Check sheet for the drawn part. Datum: minimum x, y, z corner. Units: mm. A direction names the side the tool comes from. Coordinates: 2 decimals unless noted, no trailing zeros. Loops run counter-clockwise (first coordinate to the right, second up) from the corner with the lowest first, then second, coordinate; pieces in that order, holes last. Notation, with made-up numbers: (-23, 35) -> (-15, 35) arc R11 cw to (-15, 51) -> close; hole circle Ø8 at (41.5, 70.5). An arc over 180 degrees is marked (long way). Use CSV: the item, a comma, the result in double quotes. Start each with the question number.
1. Thickness scan on L1, parallel to Z at x = 54.5, y = 2.55; L2, parallel to X at y = 4.35, z = 31; L3, parallel to X at y = 2.9, z = 48. Record the ranges inside material, lowest first.
2. Sectioned sample at A-A, the plane x = 32.3. Record the cut outline in (y, z).
3. Set-up check for the marked faces 1, 2 and 3: record each of +Z, -Z, +X, -X, +Y, -Y from which the full face is reachable in a straight line by a thin tool's end or side.
4. Sectioned sample at B-B, the plane x = 54.5. Record the cut outline in (y, z).
5. Sectioned sample at D-D, the plane z = 12.5. Record the cut outline in (x, y).
6. Gauge pin test, flat ends, axial feed: pin 1 (2 mm diameter, centred on x = 48, y = 1, fed in from -Z); pin 2 (3 mm diameter, centred on x = 12.5, y = 2, fed in from +Z); pin 3 (1 mm diameter, centred on y = 4, z = 15, fed in from -X). Record the tip position at first contact, or that the pin passes through.
7. Sectioned sample at C-C, the plane y = 3.7. Record the cut outline in (x, z).
8. Release check for a two-part mould opening along Z. For the marked faces 4, 5 and 6 record: pulls with the +Z half, pulls with the -Z half, needs draft (parallel to the pull), parting line crosses it, or undercut.
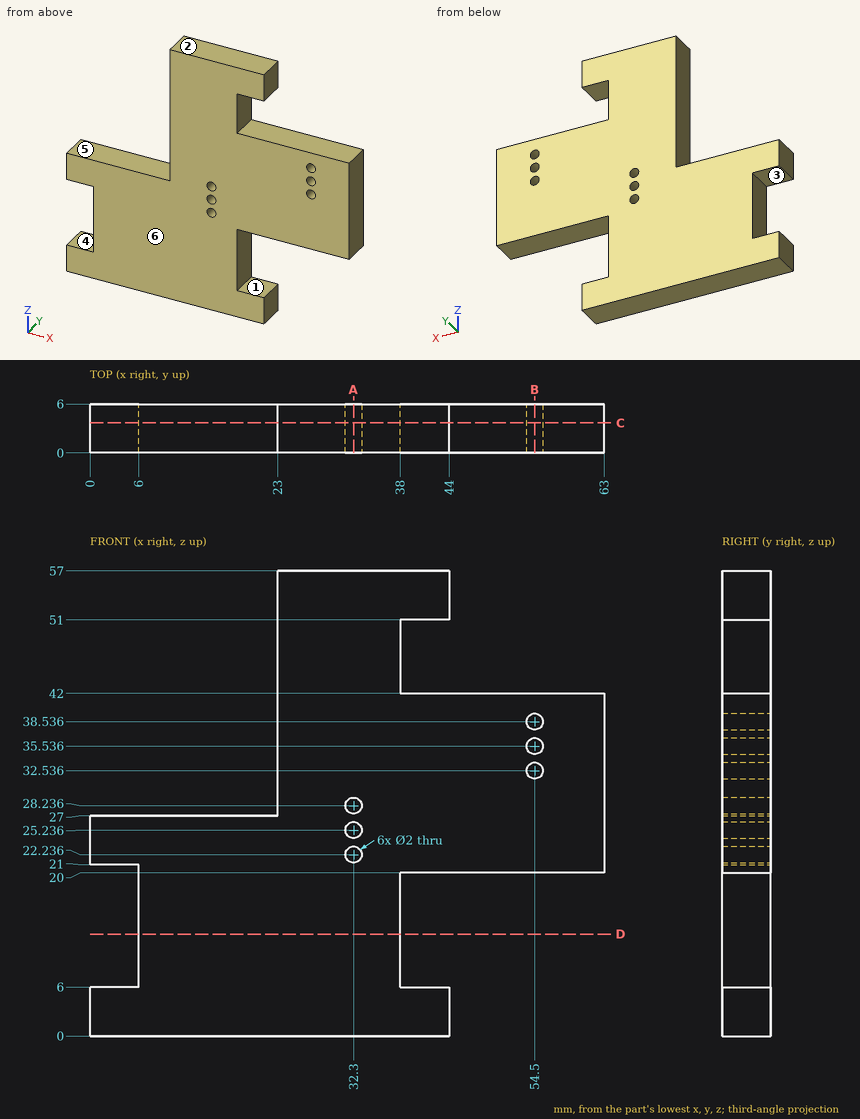
Completed:
1,L1,"20 to 31.54, 33.54 to 34.54, 36.54 to 37.54, 39.54 to 42"
1,L2,"23 to 63"
1,L3,"23 to 38"
2,outline,"(0, 0) -> (6, 0) -> (6, 21.24) -> (0, 21.24) -> close; (0, 23.24) -> (6, 23.24) -> (6, 24.24) -> (0, 24.24) -> close; (0, 26.24) -> (6, 26.24) -> (6, 27.24) -> (0, 27.24) -> close; (0, 29.24) -> (6, 29.24) -> (6, 57) -> (0, 57) -> close"
3,face 1,"+X, +Y, -Y"
3,face 2,"+Z, +X, -X, +Y, -Y"
3,face 3,"-X, +Y, -Y"
4,outline,"(0, 20) -> (6, 20) -> (6, 31.54) -> (0, 31.54) -> close; (0, 33.54) -> (6, 33.54) -> (6, 34.54) -> (0, 34.54) -> close; (0, 36.54) -> (6, 36.54) -> (6, 37.54) -> (0, 37.54) -> close; (0, 39.54) -> (6, 39.54) -> (6, 42) -> (0, 42) -> close"
5,outline,"(6, 0) -> (38, 0) -> (38, 6) -> (6, 6) -> close"
6,pin 1,"z = 20"
6,pin 2,"z = 27"
6,pin 3,"x = 6"
7,outline,"(0, 0) -> (44, 0) -> (44, 6) -> (38, 6) -> (38, 20) -> (63, 20) -> (63, 42) -> (38, 42) -> (38, 51) -> (44, 51) -> (44, 57) -> (23, 57) -> (23, 27) -> (0, 27) -> (0, 21) -> (6, 21) -> (6, 6) -> (0, 6) -> close; hole circle Ø2 at (32.3, 22.24); hole circle Ø2 at (32.3, 25.24); hole circle Ø2 at (32.3, 28.24); hole circle Ø2 at (54.5, 32.54); hole circle Ø2 at (54.5, 35.54); hole circle Ø2 at (54.5, 38.54)"
8,face 4,"undercut"
8,face 5,"pulls with the +Z half"
8,face 6,"needs draft"
